Can you work these out from the model? Positions are in its coordinate system, mm. Round coordinates to 2 decimals unless told otherwise and drop trailing zeros. Order: outer loops, then holes, each group sorted by start corner. A loop starts at its lowest first (then second) coordinate and runs counter-clockwise, first axis right, second up. Notation, with made-up numbers: M 49.5,36.25 L 57.5,36.25 A23 ccw 57.5,44.25 Z; hole C 46,59 d10. An arc over 180 degrees is marked long. Answer as a JSON object with one key per item and string values. Group by question number.
```python
from build123d import *

# Parameters (mm, degrees)
SKETCH1_R           = 3.3
BOSS_EXTRUDE1_DEPTH = 4


with BuildPart() as part:
    # Sketch1 → Boss-Extrude1 (new body)
    with BuildSketch(Plane.XY):
        with BuildLine():
            Line((5.288922953, 41.473211764), (10.211865104, 80.076576605))
            ThreePointArc((10.211865104, 80.076576605), (12.403300333, 83.154463495), (16.179730642, 83.034671229))
            Line((16.179730642, 83.034671229), (63.820269358, 55.529393377))
            ThreePointArc((63.820269358, 55.529393377), (65.683972663, 53.100567942), (65.284370973, 50.065291762))
            Line((65.284370973, 50.065291762), (53.908491826, 30.361691097))
            ThreePointArc((53.908491826, 30.361691097), (53.374672591, 28.490644117), (53.786806351, 26.589085404))
            ThreePointArc((53.786806351, 26.589085404), (60, 0), (53.786806351, -26.589085404))
            ThreePointArc((53.786806351, -26.589085404), (53.374672591, -28.490644117), (53.908491826, -30.361691097))
            Line((53.908491826, -30.361691097), (65.284370973, -50.065291762))
            ThreePointArc((65.284370973, -50.065291762), (65.683972663, -53.100567942), (63.820269358, -55.529393377))
            Line((63.820269358, -55.529393377), (16.179730642, -83.034671229))
            ThreePointArc((16.179730642, -83.034671229), (12.403300333, -83.154463495), (10.211865104, -80.076576605))
            Line((10.211865104, -80.076576605), (5.288922953, -41.473211764))
            ThreePointArc((5.288922953, -41.473211764), (5.980180313, -38.672899027), (8.375189586, -37.065566222))
            ThreePointArc((8.375189586, -37.065566222), (38, 0), (8.375189586, 37.065566222))
            ThreePointArc((8.375189586, 37.065566222), (5.980180313, 38.672899027), (5.288922953, 41.473211764))
        make_face()
        with Locations((30.329719018, 41.74527691)):
            Circle(SKETCH1_R, mode=Mode.SUBTRACT)
        with Locations((49.074516241, 15.94527691)):
            Circle(SKETCH1_R, mode=Mode.SUBTRACT)
        with Locations((49.074516241, -15.94527691)):
            Circle(SKETCH1_R, mode=Mode.SUBTRACT)
        with Locations((30.329719018, -41.74527691)):
            Circle(SKETCH1_R, mode=Mode.SUBTRACT)
        with Locations((21.009618943, 66.389727457)):
            Circle(SKETCH1_R, mode=Mode.SUBTRACT)
        with Locations((46.990381057, 51.389727457)):
            Circle(SKETCH1_R, mode=Mode.SUBTRACT)
        with Locations(Location((46.990381057, -51.389727457, 0), (0, 0, 180))):
            Circle(SKETCH1_R, mode=Mode.SUBTRACT)
        with Locations(Location((21.009618943, -66.389727457, 0), (0, 0, 180))):
            Circle(SKETCH1_R, mode=Mode.SUBTRACT)
    extrude(amount=BOSS_EXTRUDE1_DEPTH)


solid = part.part
```
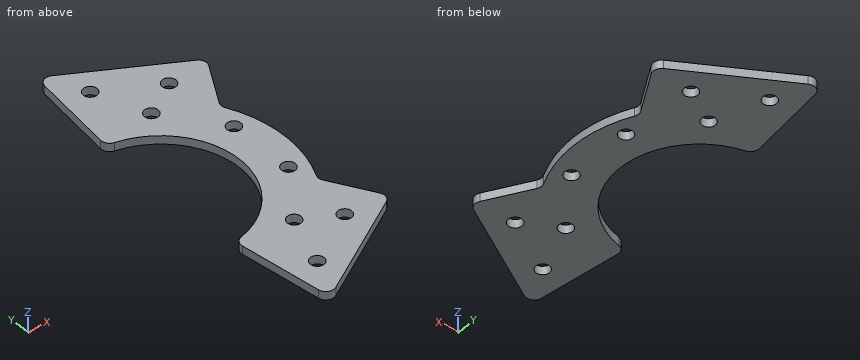
1) If we section it at D-D on y = -5.5: Write out the boundary of the cut face in (x, z), plus the area to 3 significant figures.
2) I need wall thicknesses on line 1 along Y through (x, z) = (45, 3.35); line 2 along Y through (x, z) = (23, 3.05); line 3 along Y through (x, z) = (54.5, 2.4). Which ranges of each line are inside material? Lowest first, please.
3) For pin 1 (6 mm diameter, centred on x = 46.99, y = 51.39, fed in from +Z); pin 2 (6 mm diameter, centred on x = 30, y = 30.5, fed in from -Z); pin 3 (1 mm diameter, centred on x = 12, z = 2, fed in from -Y); pin 4 (1.5 mm diameter, centred on y = 10.5, z = 2.5, fed in from +X), each with a flat end and sliding along its axis, tell me the tip position at first contact or that it passes through.
4) If we section it at C-C on z = 1.1: Count the separate pieces of the cut face and the enclosed holes in it, plus the area to 3 significant figures.
5) If we section it at B-B on x = 13: Write out the boundary of the cut face in (y, z), plus the area to 3 significant figures.
6) If we section it at A-A on x = 57: Write out the boundary of the cut face in (y, z) (3 decimals).
Findings:
{
 "1": {"outline": "M 37.6,0 L 59.75,0 L 59.75,4 L 37.6,4 Z", "area": "88.6 mm^2"},
 "2": {"line 1": "y = -66.4 to -54.02, -48.76 to 48.76, 54.02 to 66.4", "line 2": "y = -79.1 to -69.02, -63.76 to -30.25, 30.25 to 63.76, 69.02 to 79.1", "line 3": "y = -60.91 to -31.39, -25.09 to 25.09, 31.39 to 60.91"},
 "3": {"pin 1": "passes through", "pin 2": "stops at z = 0", "pin 3": "stops at y = -83.2", "pin 4": "stops at x = 59.2"},
 "4": {"separate pieces": "1", "enclosed holes": "8", "area": "5,510 mm^2"},
 "5": {"outline": "M -83.39,0 L -35.71,0 L -35.71,4 L -83.39,4 Z; M 35.71,0 L 83.39,0 L 83.39,4 L 35.71,4 Z", "area": "381 mm^2"},
 "6": {"outline": "M -59.467,0 L -35.716,0 L -35.716,4 L -59.467,4 Z; M -18.735,0 L 18.735,0 L 18.735,4 L -18.735,4 Z; M 35.716,0 L 59.467,0 L 59.467,4 L 35.716,4 Z"}
}
